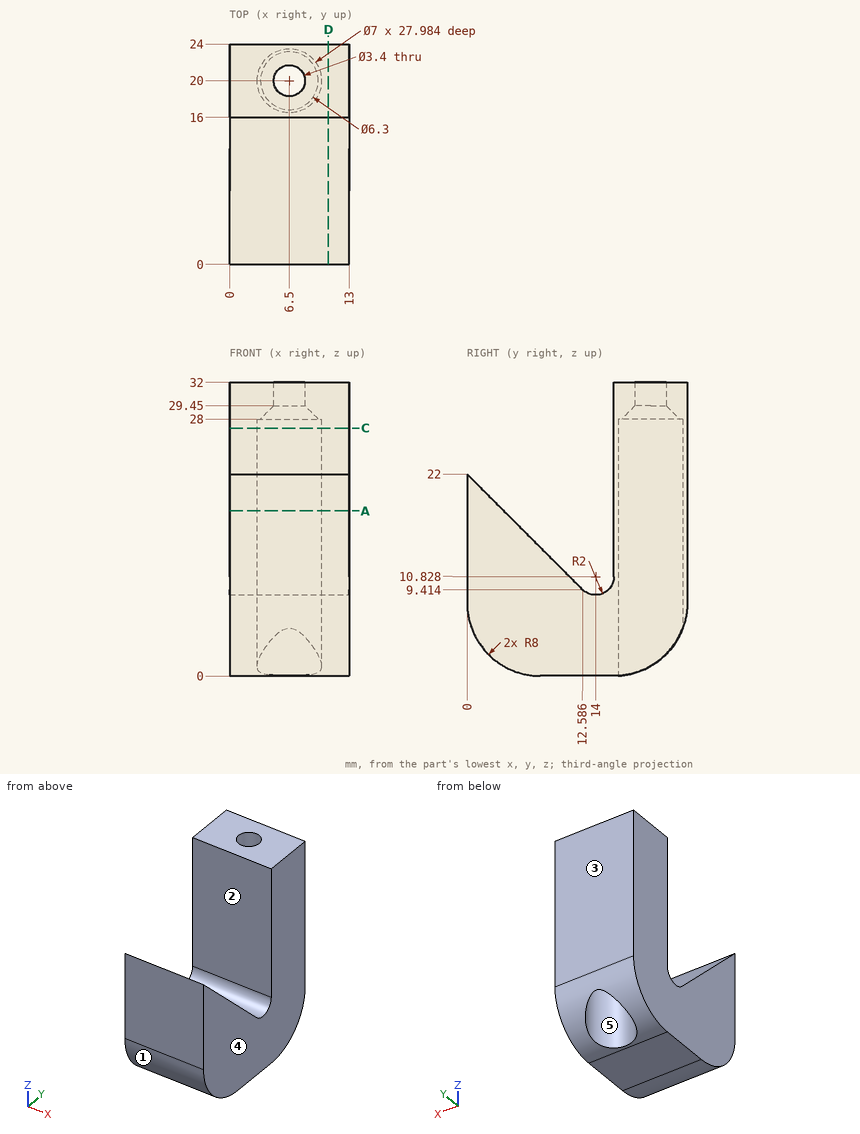
Print and shaded views of the part. All mm, measured from the part's lowest x, y and z. A direction names the side the tool comes from. Round coordinates to 2 decimals unless told otherwise and drop trailing zeros. Write each loop counter-clockwise with the first axis right and the second up, starting at its lowest first coordinate (ties: lowest second). Pieces come first, ordered by that corner, then holes.
(1) Drop flat-ended pins along their axis: P1, Ø5.5, axis at x = 6, y = 19, coming from the -Z side; P2, Ø1.5, axis at x = 11, y = 10, coming from the +Z side; P3, Ø1.5, axis at x = 10, y = 15.5, coming from the +Z side; P4, Ø4.5, axis at x = 6.5, y = 20, coming from the -Z side. Give the stop position or say it passes through.
(2) Slice it at C-C, the plane z = 27. Write the cut outline in (x, y).
(3) 3-axis set-ups, long thin cutter, end or side, ignore diameter. For the marked faces 1 and 2: which of +Z, -Z, +X, -X, +Y, -Y reach the whole face in a straight line?
(4) Slice it at D-D, the plane x = 10.75. Write the cut outline in (y, z) (1 decimal).
(5) Mould opens along X. For the marked faces 3, 4 and 5 say: pulls with the +X half, pulls with the -X half, needs draft (parallel to the pull), parting line crosses it, or undercut.
(6) Slice it at A-A, the plane z = 18. Write the cut outline in (x, y).
(7) Probe line 1 along Y through (x, z) = (6.5, 30.7); line 2 along Y through (x, z) = (5.5, 17.5) (1 decimal); line 3 along X through (y, z) = (20, 16.5). List the from-to ranges inside material, lowest first.
From the geometry:
1. P1: stops at z = 0
1. P2: stops at z = 12.75
1. P3: stops at z = 32
1. P4: stops at z = 28.9
2. outline: (0, 16) - (13, 16) - (13, 24) - (0, 24) - close; hole circle Ø7 at (6.5, 20)
3. face 1: -Z, +X, -X, -Y
3. face 2: +Z, +X, -X
4. outline: (0, 8) arc R8 ccw to (8, 0) - (16, 0) arc R8 ccw to (24, 8) - (24, 32) - (16, 32) - (16, 10.8) arc R2 cw to (12.6, 9.4) - (0, 22) - close
5. face 3: needs draft
5. face 4: pulls with the +X half
5. face 5: undercut
6. outline: (0, 0) - (13, 0) - (13, 4) - (0, 4) - close; (0, 16) - (13, 16) - (13, 24) - (0, 24) - close; hole circle Ø7 at (6.5, 20)
7. line 1: y = 16 to 18.3, 21.7 to 24
7. line 2: y = 0 to 4.5, 16 to 16.6, 23.4 to 24
7. line 3: x = 0 to 3, 10 to 13
